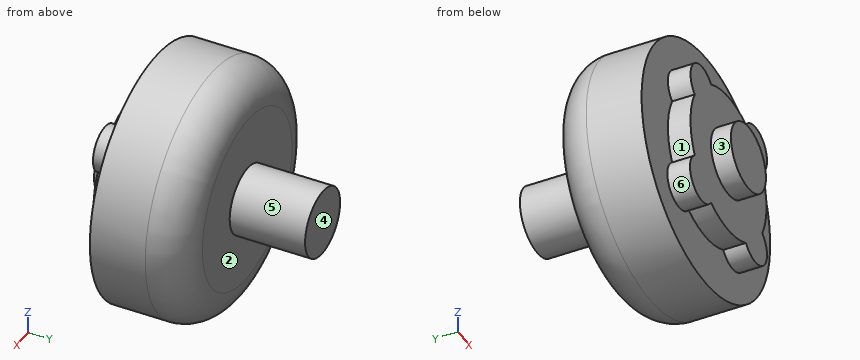
```python
from build123d import *

# Parameters (mm, degrees)
SKETCH1_W                = 16.518614554
SKETCH1_H                = 12.353050884
BOSS_EXTRUDE1_DEPTH      = 10
BOSS_EXTRUDE1_DEPTH_BACK = 18
SKETCH3_R                = 4.5
FILLET1_R                = 5
SKETCH4_R                = 9.759449404
SKETCH4_R_2              = 3
BOSS_EXTRUDE2_DEPTH      = 3
SCALE2_SCALE             = 1.5
SCALE3_SCALE             = 0.7


with BuildPart() as part:
    # Sketch1 → Revolve1 (revolve)
    with BuildSketch(Plane.XY, mode=Mode.PRIVATE) as revolve1_sk:
        with Locations((8.259307277, 6.176525442)):
            Rectangle(SKETCH1_W, SKETCH1_H)
    revolve(revolve1_sk.sketch.rotate(Axis((16.518614554, 0, 0), (0, 1, 0)), 270), axis=Axis((16.518614554, 0, 0), (0, 1, 0)))

    # Sketch3 → Boss-Extrude1 (add, two sides: drawn at the far end of the back side and taken through both)
    with BuildSketch(Plane(origin=(0, 12.353050884, 0), x_dir=(1, 0, 0), z_dir=(0, 1, 0)).offset(-BOSS_EXTRUDE1_DEPTH_BACK)):
        with Locations(Location((16.518614554, 0, 0), (0, 0, 270))):
            Circle(SKETCH3_R)
    extrude(amount=BOSS_EXTRUDE1_DEPTH + BOSS_EXTRUDE1_DEPTH_BACK)

    # Fillet1
    fillet1_edges = [part.edges().sort_by_distance(p)[0] for p in [
        (16.518614554, 12.353050884, 16.518614554),
    ]]
    fillet(fillet1_edges, radius=FILLET1_R)

    # Sketch4 → Boss-Extrude2 (add)
    with BuildSketch(Plane.XZ):
        with BuildLine():
            Line((11.738962044, -4.77965251), (16.518614554, 0))
            Line((16.518614554, 0), (11.881429434, 4.637185121))
            ThreePointArc((11.881429434, 4.637185121), (9.893846238, 3.761487884), (7.836164974, 4.456671622))
            ThreePointArc((7.836164974, 4.456671622), (6.759173098, -0.012454385), (7.847567883, -4.478817062))
            ThreePointArc((7.847567883, -4.478817062), (9.848875397, -3.909897633), (11.738962044, -4.77965251))
        make_face()
        with BuildLine():
            Line((21.298267065, 4.77965251), (16.518614554, 0))
            Line((16.518614554, 0), (21.298267065, -4.77965251))
            ThreePointArc((21.298267065, -4.77965251), (23.188353712, -3.909897633), (25.189661226, -4.478817062))
            ThreePointArc((25.189661226, -4.478817062), (26.002060498, -2.304583627), (26.278063958, 0))
            ThreePointArc((26.278063958, 0), (26.002060498, 2.304583627), (25.189661226, 4.478817062))
            ThreePointArc((25.189661226, 4.478817062), (23.188353712, 3.909897633), (21.298267065, 4.77965251))
        make_face()
        with BuildLine():
            Line((11.881429434, 4.637185121), (16.518614554, 0))
            Line((16.518614554, 0), (21.298267065, 4.77965251))
            ThreePointArc((21.298267065, 4.77965251), (20.428512187, 6.669739158), (20.997431617, 8.671046672))
            ThreePointArc((20.997431617, 8.671046672), (16.53106894, 9.759441457), (12.061942933, 8.68244958))
            ThreePointArc((12.061942933, 8.68244958), (12.580171282, 7.781857425), (12.76010909, 6.758505464))
            ThreePointArc((12.76010909, 6.758505464), (12.531747688, 5.610455167), (11.881429434, 4.637185121))
        make_face()
        with BuildLine():
            Line((21.298267065, -4.77965251), (16.518614554, 0))
            Line((16.518614554, 0), (11.738962044, -4.77965251))
            ThreePointArc((11.738962044, -4.77965251), (12.389280298, -5.752922557), (12.6176417, -6.900972854))
            ThreePointArc((12.6176417, -6.900972854), (12.469524182, -7.831975707), (12.039797492, -8.671046672))
            ThreePointArc((12.039797492, -8.671046672), (16.518614554, -9.759449404), (20.997431617, -8.671046672))
            ThreePointArc((20.997431617, -8.671046672), (20.428512187, -6.669739158), (21.298267065, -4.77965251))
        make_face()
        with Locations((16.518614554, 0)):
            Circle(SKETCH4_R)
        with Locations((9.6176417, -6.900972854)):
            Circle(SKETCH4_R_2)
        with BuildLine():
            ThreePointArc((12.6176417, -6.900972854), (12.389280298, -5.752922557), (11.738962044, -4.77965251))
            Line((11.738962044, -4.77965251), (9.6176417, -6.900972854))
            ThreePointArc((9.6176417, -6.900972854), (10.760299266, -7.879635632), (12.039797492, -8.671046672))
            ThreePointArc((12.039797492, -8.671046672), (12.469524182, -7.831975707), (12.6176417, -6.900972854))
        make_face()
        with BuildLine():
            Line((9.6176417, -6.900972854), (11.738962044, -4.77965251))
            ThreePointArc((11.738962044, -4.77965251), (9.848875397, -3.909897633), (7.847567883, -4.478817062))
            ThreePointArc((7.847567883, -4.478817062), (8.638978922, -5.758315289), (9.6176417, -6.900972854))
        make_face()
        with Locations((9.76010909, 6.758505464)):
            Circle(SKETCH4_R_2)
        with BuildLine():
            Line((11.881429434, 4.637185121), (13.336634039, 3.181980515))
            ThreePointArc((13.336634039, 3.181980515), (16.518614554, 4.5), (19.70059507, 3.181980515))
            Line((19.70059507, 3.181980515), (21.298267065, 4.77965251))
            ThreePointArc((21.298267065, 4.77965251), (20.428512187, 6.669739158), (20.997431617, 8.671046672))
            ThreePointArc((20.997431617, 8.671046672), (16.53106894, 9.759441457), (12.061942933, 8.68244958))
            ThreePointArc((12.061942933, 8.68244958), (12.580171282, 7.781857425), (12.76010909, 6.758505464))
            ThreePointArc((12.76010909, 6.758505464), (12.531747688, 5.610455167), (11.881429434, 4.637185121))
        make_face()
        with Locations((23.419587408, 6.900972854)):
            Circle(SKETCH4_R_2)
        with BuildLine():
            Line((23.419587408, 6.900972854), (21.298267065, 4.77965251))
            ThreePointArc((21.298267065, 4.77965251), (23.188353712, 3.909897633), (25.189661226, 4.478817062))
            ThreePointArc((25.189661226, 4.478817062), (24.398250187, 5.758315289), (23.419587408, 6.900972854))
        make_face()
        with BuildLine():
            ThreePointArc((20.997431617, 8.671046672), (20.428512187, 6.669739158), (21.298267065, 4.77965251))
            Line((21.298267065, 4.77965251), (23.419587408, 6.900972854))
            ThreePointArc((23.419587408, 6.900972854), (22.276929843, 7.879635632), (20.997431617, 8.671046672))
        make_face()
        with Locations((23.419587408, -6.900972854)):
            Circle(SKETCH4_R_2)
        with BuildLine():
            Line((23.419587408, -6.900972854), (21.298267065, -4.77965251))
            ThreePointArc((21.298267065, -4.77965251), (20.428512187, -6.669739158), (20.997431617, -8.671046672))
            ThreePointArc((20.997431617, -8.671046672), (22.276929843, -7.879635632), (23.419587408, -6.900972854))
        make_face()
        with BuildLine():
            ThreePointArc((25.189661226, -4.478817062), (23.188353712, -3.909897633), (21.298267065, -4.77965251))
            Line((21.298267065, -4.77965251), (23.419587408, -6.900972854))
            ThreePointArc((23.419587408, -6.900972854), (24.398250187, -5.758315289), (25.189661226, -4.478817062))
        make_face()
    extrude(amount=BOSS_EXTRUDE2_DEPTH)


with BuildPart() as part_1:
    # Scale2: scaled about (16.521177645, 5.714728263, -0.002563091)
    add(part.part.scale(SCALE2_SCALE).moved(Location((-8.260588823, -2.857364131, 0.001281545))))


with BuildPart() as part_2:
    # Scale3: scaled about (16.521177645, 5.714728263, -0.002563091)
    add(part_1.part.scale(SCALE3_SCALE).moved(Location((4.956353294, 1.714418479, -0.000768927))))


solid = part_2.part
```
The model under review builds one solid part; all positions refer to its coordinate system, in mm. Face numbers are marked on the shaded views. A direction names the side the tool comes from. Round coordinates to 2 decimals unless told otherwise and drop trailing zeros. Loops run counter-clockwise (first coordinate to the right, second up) from the corner with the lowest first, then second, coordinate; pieces in that order, holes last. Notation, with made-up numbers: (55, -16.5) - (95, -16.5) arc R29 cw to (95, 15.5) - close; hole circle Ø4 at (75.5, -33). An arc over 180 degrees is marked (long way). Use a Markdown table: item, result. Add a question column.
Q1. Insertion check: pin 1 Ø5 at (y, z) = (4.5, -4) entering from -X; pin 2 Ø8 at (x, y) = (25.5, 7) entering from +Z; pin 3 Ø4 at (x, z) = (17.5, -9.5) entering from +Y. Each pin has a flat end and moves straight along its axis. Give the tip position at first contact, or say it passes through.
Q2. The part is to be moulded in two halves that separate along X. For the marked faces 4, 5 and 6, say which applies: pulls with the +X half, pulls with the -X half, needs draft (parallel to the pull), parting line crosses it, or undercut.
Q3. Add section B-B (y = 4.75). State the section outline as (x, z) points.
Q4. For probe 1 along Y at (x, z) = (11, -8); probe 2 along X at (y, z) = (13.75, -0.5); probe 3 along X at (y, z) = (4, -8), list the stretches that pass through material, from the lowest coordinate up.
Q5. Add section A-A (y = 8). State the section outline as (x, z) points.
Q6. Machinability: for the marked faces 1, 2 and 3, which of the approach directions +Z, -Z, +X, -X, +Y, -Y give a long, thin tool a straight path to every point of the face, cutting with its end or side? Answer none if there is none.
Worked answers:
| question | item | result |
|---|---|---|
| 1 | pin 1 | x = -0.76 |
| 1 | pin 2 | z = 16.61 |
| 1 | pin 3 | y = 12.68 |
| 2 | face 4 | needs draft |
| 2 | face 5 | parting line crosses it |
| 2 | face 6 | undercut |
| 3 | outline | circle Ø34.69 at (16.52, 0) |
| 4 | probe 1 | -3.44 to 12.68 |
| 4 | probe 2 | 11.82 to 21.22 |
| 4 | probe 3 | 1.13 to 31.91 |
| 5 | outline | circle Ø34.63 at (16.52, 0) |
| 6 | face 1 | -X, -Y |
| 6 | face 2 | +Y |
| 6 | face 3 | -Y |
